Input: part model. Units: mm. Frame: model coordinates. Give positions to 0.01 mm unless a question says otherwise; leave off trailing zeros. Order: outer loops, then holes, each group sorted by start corner. A loop starts at its lowest first (then second) coordinate and runs counter-clockwise, first axis right, second up. Notation, with made-up numbers: (30.25, -5) - (74.25, -5) arc R12 ccw to (74.25, 11) - close; hole circle Ø9 at (89, 56.5). An arc over 180 degrees is marked (long way). Answer in a Markdown table with one row per item. Add a question column.
1. Ray query, line 1 (Y direction, x = 27, z = 2.7) (3 decimals); line 2 (Y direction, x = 23.5, z = 1.45) (3 decimals); line 3 (Y direction, x = 40, z = 2.75). Return the intervals inside material, ascending. Write a range as [from, to].
2. Contact query for a flat-ended pin moving along its axis: pin 1 (4 mm diameter, centred on x = 25.4, y = 246.17, fed in from +Z). Output: stop coordinate, or through.
3. Section query B-B on z = 1.1. Count the separate pieces of the cut face and the enclosed holes in it, and give its area (3 significant figures).
4. Section query A-A on y = 19.05. Return loops of the section in (x, z) (3 decimals), and give its area (3 significant figures).
Autodesk Inventor part; units mm, degrees
ref_plane "YZ Plane" through (0, 0, 0) normal (1, 0, 0) x (0, 1, 0)
ref_plane "XZ Plane" through (0, 0, 0) normal (0, 1, 0) x (-1, 0, 0)
ref_plane "XY Plane" through (0, 0, 0) normal (0, 0, 1) x (1, 0, 0)
sketch "Sketch1" plane through (0, 0, 0) normal (0, 0, 1) x (1, 0, 0)
  line L0 (0, 0) -> (50.8, 0)
  line L1 (50.8, 0) -> (50.8, 27.1979)
  line L2 (50.8, 139.7) -> (0, 139.7) construction
  line L3 (0, 139.7) -> (0, 0)
  line L4 (128.6063, 161.9886) -> (104.1161, 68.3618)
  line L5 (418.4795, 73.9788) -> (-1.9313, 310.0684)
  arc A0 (104.1161, 68.3618) -> (50.8, 27.1979) centre (93.3487, 27.1979) ccw construction
  line L6 (128.6063, 161.9886) -> (145.6601, 227.1856)
  line L7 (63.1831, 62.4318) -> (91.6427, 171.2335) construction
  arc A1 (50.8, 139.7) -> (91.6427, 171.2335) centre (50.8, 181.9168) ccw
  line L8 (95.8188, 187.1988) -> (111.3222, 246.4687)
  line L9 (91.6427, 171.2335) -> (95.8188, 187.1988)
  line L10 (50.8, 27.1979) -> (50.8, 139.7)
  line L11 (417.0097, 172.2938) -> (-48.9451, 294.1693)
  line L12 (50.8, 139.7) -> (50.8, 268.0799)
  line L13 (50.8, 268.0799) -> (0, 268.0799)
  line L14 (0, 268.0799) -> (0, 139.7)
  dimension "d0" = 50.8
  dimension "d1" = 139.7
extrude "Plate1" add sketch "Sketch1" along normal blind 3.048 contours L3 L14 L13 L12 L10 L1 L0
fillet "Corner Round2" radius 12.7 2 edges at (50.8, 0, 1.524) (0, 0, 1.524)
sketch "Sketch2" plane through (0, 0, 0) normal (0, 0, -1) x (-1, 0, 0)
  arc A0 (-20.4, 99.125) -> (-20.4, 123.125) centre (-25.4, 111.125) ccw
  line L0 (-20.4, 123.125) -> (-30.4, 123.125)
  line L1 (-30.4, 99.125) -> (-20.4, 99.125)
  arc A1 (-30.4, 123.125) -> (-30.4, 99.125) centre (-25.4, 111.125) ccw
  circle A2 centre (-13.0256, 98.7506) radius 1.65
  circle A3 centre (-37.7744, 123.4994) radius 1.65
  circle A4 centre (-13.0256, 123.4994) radius 1.65
  circle A5 centre (-37.7744, 98.7506) radius 1.65
  point P0 (0, 0)
extrude "Extrusion1" cut sketch "Sketch2" against normal up to surface (3.048 mm away)
fillet "Corner Round4" radius 25.4 2 edges at (50.8, 268.0799, 1.524) (0, 268.0799, 1.524)
sketch "Sketch6" plane through (0, 0, 3.048) normal (0, 0, 1) x (1, 0, 0)
  line L0 (406.4, 135.7009) -> (-31.623, 262.7009) construction
  circle A0 centre (25.4, 246.1677) radius 3.175
  arc A1 (50.8, 242.6799) -> (0, 242.6799) centre (25.4, 242.6799) ccw
  point P0 (0, 0)
  dimension "d33" = 6.35
  dimension "d34" = 0
extrude "Extrusion4" cut sketch "Sketch6" against normal up to next
sketch "Sketch7" plane through (0, 0, 3.048) normal (0, 0, 1) x (1, 0, 0)
  circle A0 centre (12.7, 19.05) radius 3.175
  circle A1 centre (38.1, 19.05) radius 3.175
  line L0 (38.1, 0) -> (12.7, 0)
  line L1 (0, 12.7) -> (0, 242.6799)
  line L2 (50.8, 242.6799) -> (50.8, 12.7)
  point P0 (0, 0)
  dimension "d37" = 6.35
  dimension "d38" = 6.35
  dimension "d39" = 19.05
  dimension "d40" = 12.7
  dimension "d41" = 12.7
extrude "Extrusion5" cut sketch "Sketch7" against normal up to next
equation "\"d10\" = Thickness"
equation "\"BendRadius\" = Thickness"
equation "\"BendReliefWidth\" = Thickness"
equation "\"BendReliefDepth\" = 0.5 * Thickness"
equation "\"CornerReliefSize\" = 4 * Thickness"
equation "\"MinimumRemnant\" = 2 * Thickness"
equation "\"TransitionRadius\" = BendRadius"
equation "\"JacobiRadiusSize\" = Thickness"
equation "\"GapSize\" = Thickness"
equation "\"d2\" = BendRadius"
properties part number "pG188Mount"
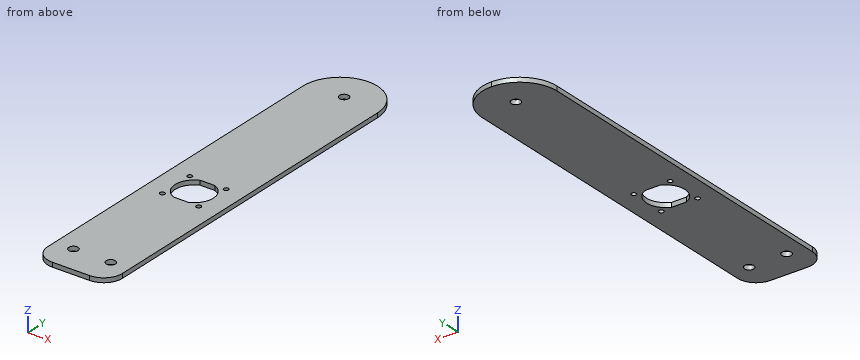
Answer:
| question | item | result |
|---|---|---|
| 1 | line 1 | y = [0, 99.125], [123.125, 243.425], [248.91, 268.029] |
| 1 | line 2 | y = [0, 99.125], [123.125, 243.624], [248.711, 268.009] |
| 1 | line 3 | y = [0.14, 16.51], [21.59, 263.46] |
| 2 | pin 1 | passes through |
| 3 | separate pieces | 1 |
| 3 | enclosed holes | 8 |
| 3 | area | 12,600 mm² |
| 4 | outline | (0, 0) - (9.525, 0) - (9.525, 3.048) - (0, 3.048) - close; (15.875, 0) - (34.925, 0) - (34.925, 3.048) - (15.875, 3.048) - close; (41.275, 0) - (50.8, 0) - (50.8, 3.048) - (41.275, 3.048) - close |
| 4 | area | 116 mm² |
